```python
from build123d import *

# Parameters (mm, degrees)
BOSS_EXTRUDE1_DEPTH = 190.5
SKETCH3_R           = 3.96875
CUT_EXTRUDE1_DEPTH  = 381
CUT_EXTRUDE2_DEPTH  = 381
SKETCH5_R           = 3.92206945
SKETCH5_R_2         = 3.96875
SKETCH5_R_3         = 3.58576203
CUT_EXTRUDE3_DEPTH  = 381
CHAMFER1_SIZE       = 25
CHAMFER1_SIZE_2     = 15
CUT_EXTRUDE4_DEPTH  = 10


with BuildPart() as part:
    # Sketch1 → Boss-Extrude1 (new, symmetric)
    with BuildSketch(Plane(origin=(0, 0, 0), x_dir=(1, 0, 0), z_dir=(0, 1, 0))):
        Polygon((-41.275, 22.225), (-41.275, -25.4), (-44.45, -25.4), (-44.45, 25.4), (44.45, 25.4), (44.45, -25.4), (41.275, -25.4), (41.275, 22.225), align=None)
    extrude(amount=BOSS_EXTRUDE1_DEPTH, both=True)

    # Sketch3 → Cut-Extrude1 (cut)
    with BuildSketch(Plane(origin=(44.45, 0, 0), x_dir=(0, 0, -1), z_dir=(1, 0, 0))):
        with Locations((0, -165.1)):
            Circle(SKETCH3_R)
    extrude(amount=-CUT_EXTRUDE1_DEPTH, mode=Mode.SUBTRACT)

    # Sketch4 → Cut-Extrude2 (cut)
    with BuildSketch(Plane(origin=(44.45, 0, 0), x_dir=(0, 0, -1), z_dir=(1, 0, 0))):
        with BuildLine():
            Line((-3.96875, -135.1), (-3.96875, -105.1))
            ThreePointArc((-3.96875, -105.1), (0, -101.13125), (3.96875, -105.1))
            Line((3.96875, -105.1), (3.96875, -135.1))
            ThreePointArc((3.96875, -135.1), (0, -139.06875), (-3.96875, -135.1))
        make_face()
        with BuildLine():
            Line((-3.96875, -54.85), (-3.96875, -24.85))
            ThreePointArc((-3.96875, -24.85), (0, -20.88125), (3.96875, -24.85))
            Line((3.96875, -24.85), (3.96875, -54.85))
            ThreePointArc((3.96875, -54.85), (0, -58.81875), (-3.96875, -54.85))
        make_face()
        with BuildLine():
            Line((-3.96875, 25.4), (-3.96875, 55.4))
            ThreePointArc((-3.96875, 55.4), (0, 59.36875), (3.96875, 55.4))
            Line((3.96875, 55.4), (3.96875, 25.4))
            ThreePointArc((3.96875, 25.4), (0, 21.43125), (-3.96875, 25.4))
        make_face()
        with BuildLine():
            Line((-3.96875, 105.65), (-3.96875, 135.65))
            ThreePointArc((-3.96875, 135.65), (0, 139.61875), (3.96875, 135.65))
            Line((3.96875, 135.65), (3.96875, 105.65))
            ThreePointArc((3.96875, 105.65), (0, 101.68125), (-3.96875, 105.65))
        make_face()
    extrude(amount=-CUT_EXTRUDE2_DEPTH, mode=Mode.SUBTRACT)

    # Sketch5 → Cut-Extrude3 (cut)
    with BuildSketch(Plane(origin=(44.45, 0, 0), x_dir=(0, 0, -1), z_dir=(1, 0, 0))):
        with Locations((0, 0.275)):
            Circle(SKETCH5_R)
        with Locations((0, -79.975)):
            Circle(SKETCH5_R_2)
        with Locations((0, 80.525)):
            Circle(SKETCH5_R_3)
        with Locations((0, 161.05)):
            Circle(SKETCH5_R_2)
    extrude(amount=-CUT_EXTRUDE3_DEPTH, mode=Mode.SUBTRACT)

    # Chamfer1
    # the kernel refuses this chamfer: 25, 15 mm, written as the material it takes off along each edge
    with BuildSketch(Plane(origin=(-109.10652743, -190.5, -25.4), x_dir=(0, -0.01989341895858275, 0.9998021063601229), z_dir=(1, 0, 0))) as chamfer1_piece_1:
        Polygon((CHAMFER1_SIZE * 0.99980210636, -CHAMFER1_SIZE * 0.0198934189586), (-CHAMFER1_SIZE_2 * 0.0198934189586, -CHAMFER1_SIZE_2 * 0.99980210636), (0, 0), align=None)
    extrude(amount=218.21305486, mode=Mode.SUBTRACT)

    # Sketch6 → Cut-Extrude4 (cut)
    with BuildSketch(Plane(origin=(0, 0, -25.4), x_dir=(-1, 0, 0), z_dir=(0, 0, -1))):
        with BuildLine():
            Line((-1.984375, -162.405), (-1.984375, -132.405))
            ThreePointArc((-1.984375, -132.405), (0, -130.420625), (1.984375, -132.405))
            Line((1.984375, -132.405), (1.984375, -162.405))
            ThreePointArc((1.984375, -162.405), (0, -164.389375), (-1.984375, -162.405))
        make_face()
        with BuildLine():
            Line((-1.984375, -112.405), (-1.984375, -82.405))
            ThreePointArc((-1.984375, -82.405), (0, -80.420625), (1.984375, -82.405))
            Line((1.984375, -82.405), (1.984375, -112.405))
            ThreePointArc((1.984375, -112.405), (0, -114.389375), (-1.984375, -112.405))
        make_face()
        with BuildLine():
            Line((-1.984375, -62.405), (-1.984375, -32.405))
            ThreePointArc((-1.984375, -32.405), (0, -30.420625), (1.984375, -32.405))
            Line((1.984375, -32.405), (1.984375, -62.405))
            ThreePointArc((1.984375, -62.405), (0, -64.389375), (-1.984375, -62.405))
        make_face()
        with BuildLine():
            Line((-2.373609799, -12.405), (-2.373609799, 17.595))
            ThreePointArc((-2.373609799, 17.595), (0, 19.968609799), (2.373609799, 17.595))
            Line((2.373609799, 17.595), (2.373609799, -12.405))
            ThreePointArc((2.373609799, -12.405), (0, -14.778609799), (-2.373609799, -12.405))
        make_face()
        with BuildLine():
            Line((-1.984375, 37.595), (-1.984375, 67.595))
            ThreePointArc((-1.984375, 67.595), (0, 69.579375), (1.984375, 67.595))
            Line((1.984375, 67.595), (1.984375, 37.595))
            ThreePointArc((1.984375, 37.595), (0, 35.610625), (-1.984375, 37.595))
        make_face()
        with BuildLine():
            Line((-1.984375, 87.595), (-1.984375, 117.595))
            ThreePointArc((-1.984375, 117.595), (0, 119.579375), (1.984375, 117.595))
            Line((1.984375, 117.595), (1.984375, 87.595))
            ThreePointArc((1.984375, 87.595), (0, 85.610625), (-1.984375, 87.595))
        make_face()
        with BuildLine():
            Line((-1.984375, 137.595), (-1.984375, 167.595))
            ThreePointArc((-1.984375, 167.595), (0, 169.579375), (1.984375, 167.595))
            Line((1.984375, 167.595), (1.984375, 137.595))
            ThreePointArc((1.984375, 137.595), (0, 135.610625), (-1.984375, 137.595))
        make_face()
        with BuildLine():
            Line((23.415625, -137.405), (23.415625, -107.405))
            ThreePointArc((23.415625, -107.405), (25.4, -105.420625), (27.384375, -107.405))
            Line((27.384375, -107.405), (27.384375, -137.405))
            ThreePointArc((27.384375, -137.405), (25.4, -139.389375), (23.415625, -137.405))
        make_face()
        with BuildLine():
            Line((23.415625, -87.405), (23.415625, -57.405))
            ThreePointArc((23.415625, -57.405), (25.4, -55.420625), (27.384375, -57.405))
            Line((27.384375, -57.405), (27.384375, -87.405))
            ThreePointArc((27.384375, -87.405), (25.4, -89.389375), (23.415625, -87.405))
        make_face()
        with BuildLine():
            Line((23.415625, -37.405), (23.415625, -7.405))
            ThreePointArc((23.415625, -7.405), (25.4, -5.420625), (27.384375, -7.405))
            Line((27.384375, -7.405), (27.384375, -37.405))
            ThreePointArc((27.384375, -37.405), (25.4, -39.389375), (23.415625, -37.405))
        make_face()
        with BuildLine():
            Line((23.415625, 12.595), (23.415625, 42.595))
            ThreePointArc((23.415625, 42.595), (25.4, 44.579375), (27.384375, 42.595))
            Line((27.384375, 42.595), (27.384375, 12.595))
            ThreePointArc((27.384375, 12.595), (25.4, 10.610625), (23.415625, 12.595))
        make_face()
        with BuildLine():
            Line((23.415625, 62.595), (23.415625, 92.595))
            ThreePointArc((23.415625, 92.595), (25.4, 94.579375), (27.384375, 92.595))
            Line((27.384375, 92.595), (27.384375, 62.595))
            ThreePointArc((27.384375, 62.595), (25.4, 60.610625), (23.415625, 62.595))
        make_face()
        with BuildLine():
            Line((23.415625, 112.595), (23.415625, 142.595))
            ThreePointArc((23.415625, 142.595), (25.4, 144.579375), (27.384375, 142.595))
            Line((27.384375, 142.595), (27.384375, 112.595))
            ThreePointArc((27.384375, 112.595), (25.4, 110.610625), (23.415625, 112.595))
        make_face()
        with BuildLine():
            Line((23.415625, 162.595), (23.415625, 182.595))
            ThreePointArc((23.415625, 182.595), (25.4, 184.579375), (27.384375, 182.595))
            Line((27.384375, 182.595), (27.384375, 162.595))
            ThreePointArc((27.384375, 162.595), (25.4, 160.610625), (23.415625, 162.595))
        make_face()
        with BuildLine():
            Line((-23.415625, -137.405), (-23.415625, -107.405))
            ThreePointArc((-23.415625, -107.405), (-25.4, -105.420625), (-27.384375, -107.405))
            Line((-27.384375, -107.405), (-27.384375, -137.405))
            ThreePointArc((-27.384375, -137.405), (-25.4, -139.389375), (-23.415625, -137.405))
        make_face()
        with BuildLine():
            Line((-23.415625, -87.405), (-23.415625, -57.405))
            ThreePointArc((-23.415625, -57.405), (-25.4, -55.420625), (-27.384375, -57.405))
            Line((-27.384375, -57.405), (-27.384375, -87.405))
            ThreePointArc((-27.384375, -87.405), (-25.4, -89.389375), (-23.415625, -87.405))
        make_face()
        with BuildLine():
            Line((-23.415625, -37.405), (-23.415625, -7.405))
            ThreePointArc((-23.415625, -7.405), (-25.4, -5.420625), (-27.384375, -7.405))
            Line((-27.384375, -7.405), (-27.384375, -37.405))
            ThreePointArc((-27.384375, -37.405), (-25.4, -39.389375), (-23.415625, -37.405))
        make_face()
        with BuildLine():
            Line((-23.415625, 12.595), (-23.415625, 42.595))
            ThreePointArc((-23.415625, 42.595), (-25.4, 44.579375), (-27.384375, 42.595))
            Line((-27.384375, 42.595), (-27.384375, 12.595))
            ThreePointArc((-27.384375, 12.595), (-25.4, 10.610625), (-23.415625, 12.595))
        make_face()
        with BuildLine():
            Line((-23.415625, 62.595), (-23.415625, 92.595))
            ThreePointArc((-23.415625, 92.595), (-25.4, 94.579375), (-27.384375, 92.595))
            Line((-27.384375, 92.595), (-27.384375, 62.595))
            ThreePointArc((-27.384375, 62.595), (-25.4, 60.610625), (-23.415625, 62.595))
        make_face()
        with BuildLine():
            Line((-23.415625, 112.595), (-23.415625, 142.595))
            ThreePointArc((-23.415625, 142.595), (-25.4, 144.579375), (-27.384375, 142.595))
            Line((-27.384375, 142.595), (-27.384375, 112.595))
            ThreePointArc((-27.384375, 112.595), (-25.4, 110.610625), (-23.415625, 112.595))
        make_face()
        with BuildLine():
            Line((-23.415625, 162.595), (-23.415625, 182.595))
            ThreePointArc((-23.415625, 182.595), (-25.4, 184.579375), (-27.384375, 182.595))
            Line((-27.384375, 182.595), (-27.384375, 162.595))
            ThreePointArc((-27.384375, 162.595), (-25.4, 160.610625), (-23.415625, 162.595))
        make_face()
    extrude(amount=-CUT_EXTRUDE4_DEPTH, mode=Mode.SUBTRACT)


solid = part.part
```
Design review of the part built by this model. Coordinates are the model's own, in mm. A direction names the side the tool comes from. Round coordinates to 2 decimals unless told otherwise and drop trailing zeros. Order: outer loops, then holes, each group sorted by start corner. A loop starts at its lowest first (then second) coordinate and runs counter-clockwise, first axis right, second up. Notation, with made-up numbers: (57.5, -6) - (106.5, -6) arc R31 ccw to (106.5, 28) - close; hole circle Ø7 at (62, 61). An arc over 180 degrees is marked (long way). Return JSON: item names as keys, results as strings.
Q1. Machinability: for faces 1 (the flat face through (-41.275, 3, -4)), 2 (the cylindrical face through (-42.84, 158.635, 3.149)), which of the approach directions +Z, -Z, +X, -X, +Y, -Y give a long, thin tool a straight path to every point of the face, cutting with its end or side? Answer none if there is none.
Computed values:
{"face 1": "+Z, +Y, -Y", "face 2": "+X, -X"}
Q2. The part is to be moulded in two halves that separate along X. For faces 3 (the flat face through (4, 190.5, -23)), 4 (the flat face through (10, 9, -22.225)), 5 (the flat face through (-44.45, 3, -5)), 6 (the flat face through (44.45, 3, 5)), say which applies: pulls with the +X half, pulls with the -X half, needs draft (parallel to the pull), parting line crosses it, or undercut.
Computed values:
{"face 3": "needs draft", "face 4": "undercut", "face 5": "pulls with the -X half", "face 6": "pulls with the +X half"}
Q3. Consider section C-C on x = 35. Write out the cut boundary in (y, z) (3 decimals), plus the area to 3 significant figures.
Computed values:
{"outline": "(-177.405, -22.225) - (-175.5, -25.4) - (190.5, -25.4) - (190.5, -22.225) - close", "area": "1,170 mm2"}
Q4. Consider section A-A on z = -9.5. Write out the cut boundary in (x, y) (3 decimals), plus the area to 3 significant figures.
Computed values:
{"outline": "(-44.45, -185.04) - (-41.275, -185.04) - (-41.275, 190.5) - (-44.45, 190.5) - close; (41.275, -185.04) - (44.45, -185.04) - (44.45, 190.5) - (41.275, 190.5) - close", "area": "2,380 mm2"}
Q5. For pin 1 Ø4 at (x, y) = (18, 129) entering from +Z (3 decimals), flat-tipped, find the tip position at first contact; note if it passes through.
Computed values:
{"pin 1": "stops at z = -22.225"}
Q6. Consider section B-B on z = 8. Write out the cut boundary in (x, y) (3 decimals).
Computed values:
{"outline": "(-44.45, -190.5) - (-41.275, -190.5) - (-41.275, 190.5) - (-44.45, 190.5) - close; (41.275, -190.5) - (44.45, -190.5) - (44.45, 190.5) - (41.275, 190.5) - close"}
Q7. Wall thickness on L1, parallel to X at y = -36, z = -9.5 (3 decimals); L2, parallel to X at y = -83.5, z = -23: over which ranges is each line inside the solid? List them lowest first. Write a range as [from, to].
Computed values:
{"L1": "x = [-44.45, -41.275], [41.275, 44.45]", "L2": "x = [-44.45, -27.38], [-23.42, -1.98], [1.98, 23.42], [27.38, 44.45]"}
